from build123d import *

# Parameters (mm, degrees)
ESQUISSE1_W        = 96
ESQUISSE1_H        = 86
BOSS_EXTRU_1_DEPTH = 5
CONG_2_R           = 5
TROUM3_D           = 3.4


with BuildPart() as part:
    # Esquisse1 → Boss.-Extru.1 (new body)
    with BuildSketch(Plane.XY):
        with Locations((2.2, -13.159463773)):
            Rectangle(ESQUISSE1_W, ESQUISSE1_H)
    extrude(amount=BOSS_EXTRU_1_DEPTH)

    # Congé2
    cong_2_edges = [part.edges().sort_by_distance(p)[0] for p in [
        (-45.8, -13.159463773, 0),
        (2.2, -56.159463773, 0),
        (50.2, -13.159463773, 0),
        (2.2, 29.840536227, 0),
    ]]
    fillet(cong_2_edges, radius=CONG_2_R - 0.0001)  # a hair under: the kernel refuses the full size

    # TrouM3 (through all)
    with Locations(Plane.XY.offset(5)):
        with Locations((-9.71, 10.960536227), (41.09, -4.279463773), (-10.98, -37.299463773), (-4.517514421, -19.876978194), (-4.517514421, -6.441949352), (8.917514421, -6.441949352), (8.917514421, -19.876978194)):
            Hole(TROUM3_D / 2)


solid = part.part
Build history of the part. All positions in model axes, mm. Round coordinates to 2 decimals unless told otherwise and drop trailing zeros. Write each loop counter-clockwise with the first axis right and the second up, starting at its lowest first coordinate (ties: lowest second). Pieces come first, ordered by that corner, then holes. Notation, with made-up numbers: (43, -13) - (94, -13) arc R29 ccw to (94, 17) - close; hole circle Ø10 at (73.5, 63.25). An arc over 180 degrees is marked (long way). One line per question, with ' | ' between items.
1. Drop flat-ended pins along their axis: pin 1 Ø2 at (x, y) = (12, -18) entering from -Z; pin 2 Ø1 at (y, z) = (13.5, 3) entering from +X. Give the stop position or say it passes through.
Results are:
pin 1: z = 0 | pin 2: x = 49.97
2. Mould opens along Y. For faces 1 (the face through (7.296, -19.366, 2.465)), 2 (the face through (2.87, 28.41, 1.5)), 3 (the face through (2, -13, 5)) say: released by +Y, released by -Y, zero draft, split by the parting line, or undercut.
Results are:
face 1: undercut | face 2: released by +Y | face 3: zero draft
3. Band-saw the part on C-C, the plane z = 1.3. Write the cut outline in (x, y), and give its area (3 significant figures).
Results are:
outline: (-44.16, -54.52) - (48.56, -54.52) - (48.56, 28.2) - (-44.16, 28.2) - close; hole circle Ø3.4 at (-10.98, -37.3); hole circle Ø3.4 at (-9.71, 10.96); hole circle Ø3.4 at (-4.52, -19.88); hole circle Ø3.4 at (-4.52, -6.44); hole circle Ø3.4 at (8.92, -19.88); hole circle Ø3.4 at (8.92, -6.44); hole circle Ø3.4 at (41.09, -4.28) | area: 7,610 mm^2
4. Drill centre lines: line 1 along Y through (x, z) = (9.5, 2); line 2 along Y through (x, z) = (-10.98, 1.3); line 3 along X through (y, z) = (-8, 1.7). Where is each one in solid material? Low to high. Write a range as from..to.
Results are:
line 1: -55.16..-21.47, -18.28..-8.04, -4.84..28.84 | line 2: -54.52..-39, -35.6..9.83, 12.09..28.2 | line 3: -44.56..-5.2, -3.84..8.24, 9.6..48.96
